Read the model definition and answer for the solid it produces. Units are mm, in the model's axes. A direction names the side the tool comes from. Round coordinates to 2 decimals unless told otherwise and drop trailing zeros. Order: outer loops, then holes, each group sorted by start corner. A loop starts at its lowest first (then second) coordinate and runs counter-clockwise, first axis right, second up. Notation, with made-up numbers: (18, 2.25) -> (27, 2.25) arc R13 cw to (27, 12.25) -> close; hole circle Ø7 at (59, -2). An arc over 180 degrees is marked (long way). One line per item, written item: value. Start each with the question number.
1. Section A-A (z = -7.95) is taken. Give the vertices of the cut face in (x, y), then the cut area to 3 significant figures.
2. The mould has two halves that part along Y. Classify faces 1 (the face through (2, -7, 0)), 2 (the face through (4, 0, 0)), 3 (the face through (2, 7, 0)), 4 (the face through (2, -15, 0)): released by +Y, released by -Y, zero draft, split by the parting line, or undercut.
3. Consider line 1 (Y direction, x = 1.55, z = -7.95); line 2 (Y direction, x = 1.7, z = -6.75); line 3 (Z direction, x = 0.95, y = 7). Determine where each line is inside the solid, lowest interval first.
4. Section B-B (x = 0.75) is taken. Give the vertices of the cut face in (y, z).
5. Section C-C (y = -11.5) is taken. Give the vertices of the cut face in (x, z).
6. For faces 5 (the face through (0.99, -2.23, -1.5)), 6 (the face through (2, 0, -10.95)), determine the directions among +Z, -Z, +X, -X, +Y, -Y from which every point of the face is accessible in a straight line to the end or side of a thin tool.
7. Flat-ended cylindrical pins translate along their axes: pin 1 Ø8 at (y, z) = (-6.5, -0.5) entering from -X; pin 2 Ø2.5 at (y, z) = (-12, -7.95) entering from +X. Find the tip coordinate at first contact, or state that the pin passes through.
8. Section D-D (x = 3.25) is taken. Give the vertices of the cut face in (y, z), then the cut area to 3 significant figures.
Autodesk Inventor part; units mm, degrees
ref_plane "YZ Plane" through (0, 0, 0) normal (1, 0, 0) x (0, 1, 0)
ref_plane "XZ Plane" through (0, 0, 0) normal (0, 1, 0) x (-1, 0, 0)
sketch "Эскиз1" plane through (0, 0, 0) normal (1, 0, 0) x (0, 1, 0)
  line L0 (-15, -10.95) -> (15, -10.95)
  line L1 (15, -10.95) -> (15, 10.95)
  line L2 (15, 10.95) -> (-15, 10.95)
  line L3 (-15, 10.95) -> (-15, -10.95)
  line L4 (-15, -10.95) -> (15, 10.95) construction
  line L5 (15, -10.95) -> (-15, 10.95) construction
  circle A0 centre (7, 0) radius 5
  circle A1 centre (-7, 0) radius 5
  point P0 (0, 0)
  dimension "d0" = 30
  dimension "d1" = 21.9
  dimension "d2" = 10
  dimension "d3" = 10
  dimension "d4" = 8
  dimension "d5" = 14
  dimension "d6" = 8
  dimension "d7" = 0
extrude "Выдавливание1" add sketch "Эскиз1" along normal blind 2
sketch "Эскиз2" plane through (2, 0, 0) normal (1, 0, 0) x (0, 0, -1)
  line L0 (10.95, 15) -> (-10.95, 15)
  line L1 (10.95, -15) -> (-10.95, -15)
  line L2 (-10.95, -15) -> (-10.95, 15)
  line L3 (-10.95, 15) -> (10.95, 15)
  line L4 (10.95, 15) -> (10.95, -15)
  line L5 (10.95, -15) -> (-10.95, 15) construction
  line L6 (-10.95, -15) -> (10.95, 15) construction
  point P0 (0, 0)
extrude "Выдавливание2" add sketch "Эскиз2" along normal blind 2
sketch "Эскиз3" plane through (0, 0, 0) normal (-1, 0, 0) x (0, 0, 1)
  circle A0 centre (-7.95, 12) radius 1.5
  line L0 (-10.95, 15) -> (10.95, 15)
  line L1 (-10.95, -15) -> (-10.95, 15)
  circle A1 centre (-7.95, -12) radius 1.5
  line L2 (10.95, -15) -> (-10.95, -15)
  circle A2 centre (7.95, 12) radius 1.5
  line L3 (10.95, 15) -> (10.95, -15)
  circle A3 centre (7.95, -12) radius 1.5
  point P0 (0, 0)
  dimension "d12" = 3
  dimension "d13" = 3
  dimension "d14" = 3
  dimension "d15" = 3
  dimension "d16" = 3
  dimension "d17" = 3
  dimension "d18" = 3
  dimension "d19" = 3
  dimension "d20" = 3
extrude "Выдавливание3" cut sketch "Эскиз3" against normal up to surface (4 mm away) contours A0 | A1 | A2 | A3
properties part number "держатель магнитов на основе"
Answer:
1. outline: (0, -15) -> (4, -15) -> (4, -13.5) -> (0, -13.5) -> close; (0, -10.5) -> (4, -10.5) -> (4, 10.5) -> (0, 10.5) -> close; (0, 13.5) -> (4, 13.5) -> (4, 15) -> (0, 15) -> close
1. area: 96.0 mm^2
2. face 1: undercut
2. face 2: zero draft
2. face 3: undercut
2. face 4: released by -Y
3. line 1: -15 to -13.5, -10.5 to 10.5, 13.5 to 15
3. line 2: -15 to -12.9, -11.1 to 11.1, 12.9 to 15
3. line 3: -10.95 to -5, 5 to 10.95
4. outline: (-15, -10.95) -> (15, -10.95) -> (15, 10.95) -> (-15, 10.95) -> close; hole circle Ø3 at (-12, -7.95); hole circle Ø3 at (-12, 7.95); hole circle Ø10 at (-7, 0); hole circle Ø10 at (7, 0); hole circle Ø3 at (12, -7.95); hole circle Ø3 at (12, 7.95)
5. outline: (0, -10.95) -> (4, -10.95) -> (4, -9.36) -> (0, -9.36) -> close; (0, -6.54) -> (4, -6.54) -> (4, 6.54) -> (0, 6.54) -> (0, 2.18) -> (2, 2.18) -> (2, -2.18) -> (0, -2.18) -> close; (0, 9.36) -> (4, 9.36) -> (4, 10.95) -> (0, 10.95) -> close
6. face 5: -X
6. face 6: -Z, +X, -X, +Y, -Y
7. pin 1: x = 2
7. pin 2: through
8. outline: (-15, -10.95) -> (15, -10.95) -> (15, 10.95) -> (-15, 10.95) -> close; hole circle Ø3 at (-12, -7.95); hole circle Ø3 at (-12, 7.95); hole circle Ø3 at (12, -7.95); hole circle Ø3 at (12, 7.95)
8. area: 629 mm^2
